from build123d import *

# Parameters (mm, degrees)
EXTRUDE_1_DEPTH = 400
FILLET_1_R      = 2


with BuildPart() as part:
    # 草图1 → 凸台-拉伸1 (new body)
    with BuildSketch(Plane.XY):
        Polygon((-2.839339828, 3.9), (2.839339828, 3.9), (5.5, 6.560660172), (5.5, 8.2), (3.1, 8.2), (3.1, 9.5), (3.6, 9.5), (3.6, 10), (7.3, 10), (10, 10), (12.7, 10), (16.4, 10), (16.4, 9.5), (16.9, 9.5), (16.9, 8.2), (14.5, 8.2), (14.5, 6.560660172), (17.160660172, 3.9), (22.839339828, 3.9), (25.5, 6.560660172), (25.5, 8.2), (23.1, 8.2), (23.1, 9.5), (23.6, 9.5), (23.6, 10), (27.3, 10), (30, 10), (32.7, 10), (36.4, 10), (36.4, 9.5), (36.9, 9.5), (36.9, 8.2), (34.5, 8.2), (34.5, 6.560660172), (37.160660172, 3.9), (42.839339828, 3.9), (45.5, 6.560660172), (45.5, 8.2), (43.1, 8.2), (43.1, 9.5), (43.6, 9.5), (43.6, 10), (47.3, 10), (50, 10), (52.7, 10), (56.4, 10), (56.4, 9.5), (56.9, 9.5), (56.9, 8.2), (54.5, 8.2), (54.5, 6.560660172), (57.160660172, 3.9), (62.839339828, 3.9), (65.5, 6.560660172), (65.5, 8.2), (63.1, 8.2), (63.1, 9.5), (63.6, 9.5), (63.6, 10), (70, 10), (70, 3.6), (69.5, 3.6), (69.5, 3.1), (68.2, 3.1), (68.2, 5.5), (66.560660172, 5.5), (63.9, 2.839339828), (63.9, -2.839339828), (66.560660172, -5.5), (68.2, -5.5), (68.2, -3.1), (69.5, -3.1), (69.5, -3.6), (70, -3.6), (70, -10), (63.6, -10), (63.6, -9.5), (63.1, -9.5), (63.1, -8.2), (65.5, -8.2), (65.5, -6.560660172), (62.839339828, -3.9), (57.160660172, -3.9), (54.5, -6.560660172), (54.5, -8.2), (56.9, -8.2), (56.9, -9.5), (56.4, -9.5), (56.4, -10), (52.7, -10), (50, -10), (47.3, -10), (43.6, -10), (43.6, -9.5), (43.1, -9.5), (43.1, -8.2), (45.5, -8.2), (45.5, -6.560660172), (42.839339828, -3.9), (37.160660172, -3.9), (34.5, -6.560660172), (34.5, -8.2), (36.9, -8.2), (36.9, -9.5), (36.4, -9.5), (36.4, -10), (32.7, -10), (30, -10), (27.3, -10), (23.6, -10), (23.6, -9.5), (23.1, -9.5), (23.1, -8.2), (25.5, -8.2), (25.5, -6.560660172), (22.839339828, -3.9), (17.160660172, -3.9), (14.5, -6.560660172), (14.5, -8.2), (16.9, -8.2), (16.9, -9.5), (16.4, -9.5), (16.4, -10), (12.7, -10), (10, -10), (7.3, -10), (3.6, -10), (3.6, -9.5), (3.1, -9.5), (3.1, -8.2), (5.5, -8.2), (5.5, -6.560660172), (2.839339828, -3.9), (-2.839339828, -3.9), (-5.5, -6.560660172), (-5.5, -8.2), (-3.1, -8.2), (-3.1, -9.5), (-3.6, -9.5), (-3.6, -10), (-10, -10), (-10, -3.6), (-9.5, -3.6), (-9.5, -3.1), (-8.2, -3.1), (-8.2, -5.5), (-6.560660172, -5.5), (-3.9, -2.839339828), (-3.9, 2.839339828), (-6.560660172, 5.5), (-8.2, 5.5), (-8.2, 3.1), (-9.5, 3.1), (-9.5, 3.6), (-10, 3.6), (-10, 10), (-3.6, 10), (-3.6, 9.5), (-3.1, 9.5), (-3.1, 8.2), (-5.5, 8.2), (-5.5, 6.560660172), align=None)
        Polygon((3.9, 2.839339828), (3.9, -2.839339828), (7.3, -6.239339828), (7.3, -8.2), (10, -8.2), (12.7, -8.2), (12.7, -6.239339828), (16.1, -2.839339828), (16.1, 2.839339828), (12.7, 6.239339828), (12.7, 8.2), (10, 8.2), (7.3, 8.2), (7.3, 6.239339828), align=None, mode=Mode.SUBTRACT)
        Polygon((23.9, 2.839339828), (23.9, -2.839339828), (27.3, -6.239339828), (27.3, -8.2), (30, -8.2), (32.7, -8.2), (32.7, -6.239339828), (36.1, -2.839339828), (36.1, 2.839339828), (32.7, 6.239339828), (32.7, 8.2), (30, 8.2), (27.3, 8.2), (27.3, 6.239339828), align=None, mode=Mode.SUBTRACT)
        Polygon((43.9, 2.839339828), (43.9, -2.839339828), (47.3, -6.239339828), (47.3, -8.2), (50, -8.2), (52.7, -8.2), (52.7, -6.239339828), (56.1, -2.839339828), (56.1, 2.839339828), (52.7, 6.239339828), (52.7, 8.2), (50, 8.2), (47.3, 8.2), (47.3, 6.239339828), align=None, mode=Mode.SUBTRACT)
    extrude(amount=EXTRUDE_1_DEPTH)

    # 圆角1
    fillet_1_edges = [part.edges().sort_by_distance(p)[0] for p in [
        (-10, 10, 200),
        (70, 10, 200),
        (70, -10, 200),
        (-10, -10, 200),
    ]]
    fillet(fillet_1_edges, radius=FILLET_1_R)


solid = part.part
Source: CAD feature listing. Evaluate the final solid. Frame: model axes, mm. Coordinates: 2 decimals unless noted, no trailing zeros. Return JSON: item names as keys, results as strings.
Q1. Material intervals for line 1 along X through (y, z) = (1.5, 246); line 2 along Y through (x, z) = (53.5, 291); line 3 along X through (y, z) = (-8.25, 20), sorted ascending.
Results:
{"line 1": "-3.9 to 3.9, 16.1 to 23.9, 36.1 to 43.9, 56.1 to 63.9", "line 2": "-10 to -5.44, 5.44 to 10", "line 3": "-9.98 to -3.1, 3.1 to 16.9, 23.1 to 36.9, 43.1 to 56.9, 63.1 to 69.98"}
Q2. Contact query for flat-ended pins moving along their axis: P1, Ø4.5, axis at x = 40.5, z = 196, coming from the +Y side; P2, Ø2, axis at x = 59.5, z = 202.5, coming from the -Y side. Output: stop coordinate, or through.
Results:
{"P1": "y = 3.9", "P2": "y = -3.9"}
Q3. Section A-A, the plane z = 370. Give the number of separate pieces and of enclosed holes in the cut face, plus the area to 3 significant figures.
Results:
{"separate pieces": "1", "enclosed holes": "3", "area": "627 mm2"}
